Check sheet for the modelled part. Datum: model origin and axes. Units: mm. A direction names the side the tool comes from. Give positions to 0.01 mm unless a question says otherwise; leave off trailing zeros. Loops run counter-clockwise (first coordinate to the right, second up) from the corner with the lowest first, then second, coordinate; pieces in that order, holes last. Notation, with made-up numbers: M -27,-29.5 L 32,-29.5 A28 ccw 32,-0.5 Z; hole C 31,78.5 d1. An arc over 180 degrees is marked long. One line per question, with ' | ' between items. Start each with the question number.
Autodesk Inventor part; units mm, degrees
ref_plane "YZ Plane" through (0, 0, 0) normal (1, 0, 0) x (0, 1, 0)
ref_plane "XZ Plane" through (0, 0, 0) normal (0, 1, 0) x (-1, 0, 0)
ref_plane "XY Plane" through (0, 0, 0) normal (0, 0, 1) x (1, 0, 0)
sketch "Skizze1" plane through (0, 0, 0) normal (1, 0, 0) x (0, 1, 0)
  circle A0 centre (0, 0) radius 20
  dimension "d0" = 40
extrude "Extrusion1" add sketch "Skizze1" along normal blind 1
sketch "Skizze2" plane through (1, 0, 0) normal (1, 0, 0) x (0, 0, -1)
  circle A0 centre (0, 0) radius 20
  circle A1 centre (0, 0) radius 17
  dimension "d3" = 34
extrude "Extrusion2" add sketch "Skizze2" along normal blind 20 contours A1
sketch "Skizze5" plane through (0, 0, 0) normal (-1, 0, 0) x (0, 0, 1)
  circle A0 centre (0, 0) radius 20
  circle A1 centre (0, 0) radius 5
  dimension "d12" = 10
extrude "Extrusion5" add sketch "Skizze5" along normal blind 10 contours A1
sketch "Skizze6" plane through (21, 0, 0) normal (1, 0, 0) x (0, 0, -1)
  circle A0 centre (0, 0) radius 17
  circle A1 centre (0, 0) radius 11.1
  dimension "d15" = 22.2
extrude "Extrusion6" cut sketch "Skizze6" against normal through all contours A1
properties part number "Rolle_schieber22.2"
Q1. Cross-section at A-A (z = 0). Record the cut outline in (x, y), and give its area (3 significant figures).
Q2. Material ranges on probe 1 along Y at (x, z) = (9, 0); probe 2 along Y at (x, z) = (2.25, 10); probe 3 along Z at (x, y) = (9.75, -1), recorded low to high. Write a range as from..to.
Q3. Access from +Z, -Z, +X, -X, +Y, -Y to the whole of each face (thin tool, end or side, straight path). Record for faces 4 (the flat face through (0, 9, -9)), 5 (the cylindrical face through (10.86, -14.334, -9.139)).
Q4. Depth check by flat-ended pin: P1, Ø4, axis at y = -13, z = 3.5, coming from the -X side; P2, Ø6, axis at x = 11.5, y = 8, coming from the -Z side; P3, Ø5, axis at x = 14.5, z = 8.5, coming from the +Y side; P4, Ø4, axis at x = 7, z = 10, coming from the -Y side. Enter the tip coordinate at first touch or a pass-through.
Q5. Draft check along Y on faces 1 (the cylindrical face through (0.493, -4.336, 19.524)), 2 (the flat face through (1, -9, -15)), 3 (the cylindrical face through (10.65, 9.36, -5.97)). Enter one of: released by +Y, released by -Y, zero draft, split by the parting line, or undercut.
Q6. Cross-section at C-C (x = 3.5). Record the cut outline in (y, z), and give its area (3 significant figures).
Solved:
1) outline: M 0,-20 L 1,-20 L 1,-17 L 21,-17 L 21,-11.1 L 0,-11.1 Z; M 0,11.1 L 21,11.1 L 21,17 L 1,17 L 1,20 L 0,20 Z | area: 254 mm²
2) probe 1: y = -17..-11.1, 11.1..17 | probe 2: y = -13.75..-4.82, 4.82..13.75 | probe 3: z = -16.97..-11.05, 11.05..16.97
3) face 4: +Z, -Z, -X, +Y, -Y | face 5: +X
4) P1: stops at x = 0 | P2: stops at z = -16.25 | P3: stops at y = 15.91 | P4: stops at y = -15
5) face 1: split by the parting line | face 2: zero draft | face 3: undercut
6) outline: C 0,0 d34; hole C 0,0 d22.2 | area: 521 mm²
